```python
from build123d import *

# Parameters (mm, degrees)
F0_R     = 3.1
F0_R_2   = 8
F0_R_3   = 10
F0_R_4   = 12
F0_R_5   = 5
F0_W     = 60
F0_H     = 80
F0_W_2   = 64.935833
F0_H_2   = 61.036522
F1_DEPTH = 4


with BuildPart() as f1:
    # F0 (on Front) → F1 (new body)
    with BuildSketch(Plane.XZ):
        Polygon((500, 90), (-500, 90), (-500, 0), (-100, 0), (100, 0), (500, 0), align=None)
        with Locations((-348, 30)):
            Circle(F0_R, mode=Mode.SUBTRACT)
        with Locations((-330, 30)):
            Circle(F0_R, mode=Mode.SUBTRACT)
        with Locations((-312, 30)):
            Circle(F0_R, mode=Mode.SUBTRACT)
        with Locations((-294, 30)):
            Circle(F0_R, mode=Mode.SUBTRACT)
        with Locations((-276, 30)):
            Circle(F0_R, mode=Mode.SUBTRACT)
        with Locations((-258, 30)):
            Circle(F0_R, mode=Mode.SUBTRACT)
        with Locations((-80, 20)):
            Circle(F0_R_2, mode=Mode.SUBTRACT)
        with Locations((-130, 25)):
            Circle(F0_R_3, mode=Mode.SUBTRACT)
        with Locations((-240, 30)):
            Circle(F0_R, mode=Mode.SUBTRACT)
        with Locations((-180, 30)):
            Circle(F0_R, mode=Mode.SUBTRACT)
        with Locations((320, 25)):
            Circle(F0_R_3, mode=Mode.SUBTRACT)
        with Locations((-460, 45)):
            Circle(F0_R_3, mode=Mode.SUBTRACT)
        with Locations((-420, 45)):
            Circle(F0_R_4, mode=Mode.SUBTRACT)
        Polygon((-392, 29.25), (-392, 60.75), (-378, 60.75), (-364, 60.75), (-364, 29.25), (-378, 29.25), align=None, mode=Mode.SUBTRACT)
        with Locations((-348, 60)):
            Circle(F0_R_5, mode=Mode.SUBTRACT)
        with Locations((-330, 60)):
            Circle(F0_R_5, mode=Mode.SUBTRACT)
        with Locations((-312, 60)):
            Circle(F0_R_5, mode=Mode.SUBTRACT)
        with Locations((-294, 60)):
            Circle(F0_R_5, mode=Mode.SUBTRACT)
        with Locations((-276, 60)):
            Circle(F0_R_5, mode=Mode.SUBTRACT)
        with Locations((-258, 60)):
            Circle(F0_R_5, mode=Mode.SUBTRACT)
        Polygon((-224, 29.25), (-224, 60.75), (-210, 60.75), (-196, 60.75), (-196, 29.25), (-210, 29.25), align=None, mode=Mode.SUBTRACT)
        with Locations((-240, 60)):
            Circle(F0_R_5, mode=Mode.SUBTRACT)
        with Locations((-180, 60)):
            Circle(F0_R_5, mode=Mode.SUBTRACT)
        with Locations((-160, 60)):
            Circle(F0_R_5, mode=Mode.SUBTRACT)
        Polygon((-95.556349, 55), (-80, 70.556349), (-64.443651, 55), (-80, 39.443651), align=None, mode=Mode.SUBTRACT)
        with Locations((-30, 55)):
            Circle(F0_R_5, mode=Mode.SUBTRACT)
        with Locations((-130, 65)):
            Circle(F0_R_3, mode=Mode.SUBTRACT)
        with Locations((154.765666, 45)):
            Rectangle(F0_W, F0_H, mode=Mode.SUBTRACT)
        with Locations((240.529969, 45)):
            Rectangle(F0_W_2, F0_H_2, mode=Mode.SUBTRACT)
        with Locations((25, 55)):
            Circle(F0_R_5, mode=Mode.SUBTRACT)
        with Locations((80, 55)):
            Circle(F0_R_5, mode=Mode.SUBTRACT)
        with Locations((320, 65)):
            Circle(F0_R_3, mode=Mode.SUBTRACT)
        with BuildLine():
            Line((100, 0), (-100, 0))
            add(Edge.make_bspline(
                [(-100, 0), (-90, 0), (-90, -20), (-80, -20)],
                knots=[0, 0, 0, 0, 28.284271, 28.284271, 28.284271, 28.284271], degree=3))
            Line((-80, -20), (80, -20))
            add(Edge.make_bspline(
                [(100, 0), (90, 0), (90, -20), (80, -20)],
                knots=[0, 0, 0, 0, 28.284271, 28.284271, 28.284271, 28.284271], degree=3))
        make_face()
    extrude(amount=F1_DEPTH)


solid = f1.part
```
Part model, mm, in its own coordinate system. A direction names the side the tool comes from. Give positions to 0.01 mm unless a question says otherwise; leave off trailing zeros. Put each result on its own line as item: value. Start each with the question number.
Item 1: Pin check, flat tips, straight feed: pin 1 Ø1.5 at (y, z) = (-2, -6.5) entering from +X; pin 2 Ø13 at (x, z) = (-80, 20) entering from +Y; pin 3 Ø1 at (x, y) = (352, -2.5) entering from -Z. Stop position of each tip, or through.
Item 2: Pull direction Z, two halves, no side cores. Call faces 3 (the face through (-140, -2, 65)), 4 (the face through (-7, 0, 48)): pulls with the +Z half, pulls with the -Z half, needs draft (parallel to the pull), parting line crosses it, or undercut.
Item 3: Cut at A-A (y = -2.75). State how many separate pieces and enclosed holes the cut face has, then the cut area to 3 significant figures.
Item 4: Which spindle directions (+Z, -Z, +X, -X, +Y, -Y) get a long thin tool onto all of the face, cutting with end or side? Do faces 1 (the face through (-87.887, -1.972, 62.669)), 2 (the face through (-7, -4, 48)). Say none if no direction does.
Item 5: Wall check: L1, parallel to Z at x = 320, y = -0.9; L2, parallel to Z at x = -276, y = -1.9; L3, parallel to Z at x = 239.5, y = -0.6. Give the ranges that are in metal, low to high. Write a range as [from, to].
Answer list:
1. pin 1: stops at x = 92.25
1. pin 2: passes through
1. pin 3: stops at z = 0
2. face 3: undercut
2. face 4: needs draft
3. separate pieces: 1
3. enclosed holes: 32
3. area: 79,200 mm2
4. face 1: +Y, -Y
4. face 2: +Z, -Z, +X, -X, -Y
5. L1: z = [0, 15], [35, 55], [75, 90]
5. L2: z = [0, 26.9], [33.1, 55], [65, 90]
5. L3: z = [0, 14.48], [75.52, 90]
